from build123d import *

# Parameters (mm, degrees)
BOSS_EXTRUDE1_DEPTH      = 6.35
BOSS_EXTRUDE1_DEPTH_BACK = 6.35
BOSS_EXTRUDE2_START      = -12.7
BOSS_EXTRUDE2_DEPTH      = 12.7
SKETCH4_R                = 28.575
CUT_EXTRUDE1_DEPTH       = 61.157662646
SKETCH5_R                = 28.575
BOSS_EXTRUDE3_DEPTH      = 6.35
F_0_257_DIAMETER_HOLE1_D = 6.5278
CUT_EXTRUDE2_DEPTH       = 94.825678832
CUT_EXTRUDE2_DEPTH_BACK  = 94.825678832
SKETCH8_W                = 12.7
SKETCH8_H                = 88.9
FILLET3_R                = 38.1
SKETCH10_R               = 1.786001
CUT_EXTRUDE4_DEPTH       = 94.17880933


with BuildPart() as part:
    # Sketch1 → Boss-Extrude1 (new, two sides: drawn at the far end of the back side and taken through both)
    with BuildSketch(Plane.XY.offset(-BOSS_EXTRUDE1_DEPTH_BACK)):
        with BuildLine():
            Line((27.49630657, 15.875), (38.494829198, 22.225))
            ThreePointArc((38.494829198, 22.225), (19.878280804, 29.537115412), (0, 31.75))
            Line((0, 31.75), (0, 44.45))
            ThreePointArc((0, 44.45), (-15.640751899, 31.983653865), (-27.49630657, 15.875))
            Line((-27.49630657, 15.875), (-38.494829198, 22.225))
            ThreePointArc((-38.494829198, 22.225), (-35.519032703, 2.446538454), (-27.49630657, -15.875))
            Line((-27.49630657, -15.875), (-38.494829198, -22.225))
            ThreePointArc((-38.494829198, -22.225), (-19.878280804, -29.537115412), (0, -31.75))
            Line((0, -31.75), (0, -44.45))
            ThreePointArc((0, -44.45), (15.640751899, -31.983653865), (27.49630657, -15.875))
            Line((27.49630657, -15.875), (38.494829198, -22.225))
            ThreePointArc((38.494829198, -22.225), (35.519032703, -2.446538454), (27.49630657, 15.875))
        make_face()
        with BuildLine():
            ThreePointArc((-11.129967969, 17.779280801), (-16.817028225, 8.924127912), (-20.962292819, -0.749194604))
            ThreePointArc((-20.962292819, -0.749194604), (-16.137035591, -10.101909703), (-9.83232485, -18.528475405))
            ThreePointArc((-9.83232485, -18.528475405), (0.679992634, -19.026037615), (11.129967969, -17.779280801))
            ThreePointArc((11.129967969, -17.779280801), (16.817028225, -8.924127912), (20.962292819, 0.749194604))
            ThreePointArc((20.962292819, 0.749194604), (16.137035591, 10.101909703), (9.83232485, 18.528475405))
            ThreePointArc((9.83232485, 18.528475405), (-0.679992634, 19.026037615), (-11.129967969, 17.779280801))
        make_face(mode=Mode.SUBTRACT)
    extrude(amount=BOSS_EXTRUDE1_DEPTH + BOSS_EXTRUDE1_DEPTH_BACK)

    # Sketch3 → Boss-Extrude2 (add)
    with BuildSketch(Plane.XY.offset(6.35).offset(BOSS_EXTRUDE2_START)):
        with BuildLine():
            ThreePointArc((-11.129967969, 17.779280801), (-16.817028225, 8.924127912), (-20.962292819, -0.749194604))
            ThreePointArc((-20.962292819, -0.749194604), (-16.137035591, -10.101909703), (-9.83232485, -18.528475405))
            ThreePointArc((-9.83232485, -18.528475405), (0.679992634, -19.026037615), (11.129967969, -17.779280801))
            ThreePointArc((11.129967969, -17.779280801), (16.817028225, -8.924127912), (20.962292819, 0.749194604))
            ThreePointArc((20.962292819, 0.749194604), (16.137035591, 10.101909703), (9.83232485, 18.528475405))
            ThreePointArc((9.83232485, 18.528475405), (-0.679992634, 19.026037615), (-11.129967969, 17.779280801))
        make_face()
    extrude(amount=BOSS_EXTRUDE2_DEPTH)

    # Sketch4 → Cut-Extrude1 (cut, through all)
    with BuildSketch(Plane.XY.offset(6.35)):
        Circle(SKETCH4_R)
    extrude(amount=-CUT_EXTRUDE1_DEPTH, mode=Mode.SUBTRACT)

    # Sketch5 → Boss-Extrude3 (add)
    with BuildSketch(Plane(origin=(0, 0, -6.35), x_dir=(-1, 0, 0), z_dir=(0, 0, -1))):
        with BuildLine():
            Line((-46.293490064, -11.011328104), (-58.217602687, -7.926026976))
            Line((-58.217602687, -7.926026976), (-65.090673557, -6.147656209))
            ThreePointArc((-65.090673557, -6.147656209), (-69.850111749, 0), (-65.090673557, 6.147656209))
            Line((-65.090673557, 6.147656209), (-46.293490064, 11.011328104))
            Line((-46.293490064, 11.011328104), (-33.653938233, 17.861199328))
            ThreePointArc((-33.653938233, 17.861199328), (-19.05, 32.995567884), (1.358716756, 38.075765111))
            Line((1.358716756, 38.075765111), (13.610655164, 45.597002477))
            Line((13.610655164, 45.597002477), (27.221310328, 59.444004954))
            ThreePointArc((27.221310328, 59.444004954), (34.925055875, 60.491971232), (37.869363229, 53.296348745))
            Line((37.869363229, 53.296348745), (32.6828349, 34.585674373))
            Line((32.6828349, 34.585674373), (32.295221476, 20.214565783))
            ThreePointArc((32.295221476, 20.214565783), (38.1, 0), (32.295221476, -20.214565783))
            Line((32.295221476, -20.214565783), (32.6828349, -34.585674373))
            Line((32.6828349, -34.585674373), (37.869363229, -53.296348745))
            ThreePointArc((37.869363229, -53.296348745), (34.925055875, -60.491971232), (27.221310328, -59.444004954))
            Line((27.221310328, -59.444004954), (13.610655164, -45.597002477))
            Line((13.610655164, -45.597002477), (1.358716756, -38.075765111))
            ThreePointArc((1.358716756, -38.075765111), (-19.05, -32.995567884), (-33.653938233, -17.861199328))
            Line((-33.653938233, -17.861199328), (-46.293490064, -11.011328104))
        make_face()
        with Locations(Location((0, 0, 0), (0, 0, 180))):
            Circle(SKETCH5_R, mode=Mode.SUBTRACT)
    extrude(amount=BOSS_EXTRUDE3_DEPTH)

    # F _0.257_ Diameter Hole1 (through all)
    with Locations(Plane.XY.offset(-6.35)):
        with Locations((-31.75, 54.99261314), (63.5, 0), (-31.75, -54.99261314), (0, 0)):
            Hole(F_0_257_DIAMETER_HOLE1_D / 2)

    # Sketch8 → Cut-Extrude2 (cut, two sides: drawn at the far end of the back side and taken through both)
    with BuildSketch(Plane(origin=(0, 0, 0), x_dir=(0, 0, -1), z_dir=(1, 0, 0)).offset(-CUT_EXTRUDE2_DEPTH_BACK)):
        Rectangle(SKETCH8_W, SKETCH8_H)
    extrude(amount=CUT_EXTRUDE2_DEPTH + CUT_EXTRUDE2_DEPTH_BACK, mode=Mode.SUBTRACT)

    # Fillet3
    fillet3_edges = [part.edges().sort_by_distance(p)[0] for p in [
        (46.293490064, -11.011328104, -9.525),
        (33.653938233, -17.861199328, -9.525),
        (-1.358716756, -38.075765111, -9.525),
        (-13.610655164, -45.597002477, -9.525),
        (-32.6828349, -34.585674373, -9.525),
        (-32.295221476, -20.214565783, -9.525),
        (-32.295221476, 20.214565783, -9.525),
        (-32.6828349, 34.585674373, -9.525),
        (-13.610655164, 45.597002477, -9.525),
        (-1.358716756, 38.075765111, -9.525),
        (33.653938233, 17.861199328, -9.525),
        (46.293490064, 11.011328104, -9.525),
    ]]
    fillet(fillet3_edges, radius=FILLET3_R)

    # Sketch10 → Cut-Extrude4 (cut, through all)
    with BuildSketch(Plane(origin=(0, 0, -12.7), x_dir=(-1, 0, 0), z_dir=(0, 0, -1))):
        with Locations((-5.788996123, 32.831028466)):
            Circle(SKETCH10_R)
        with Locations((31.327002745, -11.402096528)):
            Circle(SKETCH10_R)
        with Locations((-25.538006622, -21.428931938)):
            Circle(SKETCH10_R)
    extrude(amount=-CUT_EXTRUDE4_DEPTH, mode=Mode.SUBTRACT)


solid = part.part
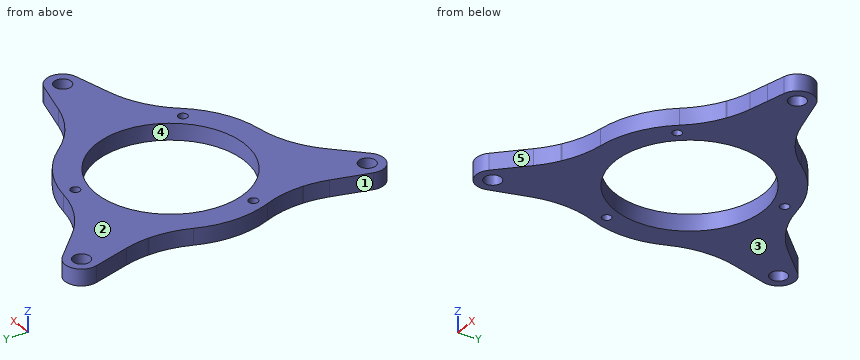
For this review, take the finished solid that the model builds, in its own axes (mm). Face numbers are marked on the shaded views. A direction names the side the tool comes from. Coordinates: 2 decimals unless noted, no trailing zeros. Order: outer loops, then holes, each group sorted by start corner. A loop starts at its lowest first (then second) coordinate and runs counter-clockwise, first axis right, second up. Notation, with made-up numbers: (21.5, 3.5) - (79.5, 3.5) arc R14 ccw to (79.5, 22.5) - close; hole circle Ø5 at (57, 38.25). An arc over 180 degrees is marked (long way). Answer as CSV lines item,"result". Start each with the question number.
1) Insertion check: P1, Ø3, axis at y = -47.5, z = -12, coming from the -X side; P2, Ø1.5, axis at y = -43.5, z = -11.5, coming from the +X side; P3, Ø2, axis at y = 16, z = -9.5, coming from the +X side. Each pin has a flat end and moves straight along its axis. Give the tip position at first contact, or say it passes through.
2) Add section A-A (y = 0). State the section outline as (x, z) points (3 decimals), then the cut area to 3 significant figures.
3) Draft analysis for pull direction Y (two halves, no side actions). For the marked faces 3, 4 and 5, state which applies: +Y half, -Y half, draft (parallel to the pull), parting line (faces both ways), or undercut.
4) Add section C-C (y = 19). State the section outline as (x, z) points.
5) Add section B-B (x = 63.5). State the section outline as (y, z) points, then the cut area to 3 significant figures.
6) Machinability: for the marked faces 1 and 2, which of the approach directions +Z, -Z, +X, -X, +Y, -Y give a long, thin tool a straight path to every point of the face, cutting with its end or side? Answer none if there is none.
7) Add section D-D (z = -10.75). Count the separate pieces of the cut face and the enclosed holes in it, then the cut area to 3 significant figures.
8) To check wall thickness, follow line 1 along X through (y, z) = (-22, -10.5); line 2 along Y through (x, z) = (-31.75, -9.75); line 3 along Y through (x, z) = (-1, -11.25). State the ranges of each line that lie inside material, in increasing order. Write a range as [from, to].
Result:
1,P1,"x = -36.68"
1,P2,"x = -8.97"
1,P3,"x = 39.21"
2,outline,"(-38.1, -12.7) - (-28.575, -12.7) - (-28.575, -6.35) - (-38.1, -6.35) - close; (28.575, -12.7) - (60.236, -12.7) - (60.236, -6.35) - (28.575, -6.35) - close; (66.764, -12.7) - (69.85, -12.7) - (69.85, -6.35) - (66.764, -6.35) - close"
2,area,"281 mm^2"
3,face 3,"draft"
3,face 4,"undercut"
3,face 5,"-Y half"
4,outline,"(-33.76, -12.7) - (-21.34, -12.7) - (-21.34, -6.35) - (-33.76, -6.35) - close; (21.34, -12.7) - (34.1, -12.7) - (34.1, -6.35) - (21.34, -6.35) - close"
5,outline,"(-6.56, -12.7) - (-3.26, -12.7) - (-3.26, -6.35) - (-6.56, -6.35) - close; (3.26, -12.7) - (6.56, -12.7) - (6.56, -6.35) - (3.26, -6.35) - close"
5,area,"41.9 mm^2"
6,face 1,"+Z, -Z, -X"
6,face 2,"+Z, +X, -X, +Y, -Y"
7,separate pieces,"1"
7,enclosed holes,"7"
7,area,"3,780 mm^2"
8,line 1,"[-33.11, -18.24], [18.24, 23.85], [27.23, 31.22]"
8,line 2,"[-61.34, -58.26], [-51.73, -13.14], [-9.67, 51.73], [58.26, 61.34]"
8,line 3,"[-39.16, -28.56], [28.56, 39.16]"
